```python
from build123d import *

# Parameters (mm, degrees)
CUT_EXTRUDE_1_REACH = 159.944
SKETCH_2_R          = 2.15


with BuildPart() as part:
    # 草图1 → 旋转1 (revolve)
    with BuildSketch(Plane.XY, mode=Mode.PRIVATE) as revolve_1_sk:
        Polygon((111.6, 6.1), (111.6, 8.1), (109.6, 8.1), (109.6, 6.1), (96.1, 6.1), (96.1, 0), (111.6, 0), align=None)
    revolve(revolve_1_sk.sketch.rotate(Axis((0, 0, 0), (0, 1, 0)), 90), axis=Axis((0, 0, 0), (0, 1, 0)))

    # 草图2 → 切除-拉伸1 (cut, up to next)
    with BuildSketch(Plane(origin=(0, 6.1, 0), x_dir=(1, 0, 0), z_dir=(0, 1, 0)), mode=Mode.PRIVATE) as cut_extrude_1_sk1:
        with Locations(Location((-100.25, 0, 0), (0, 0, 270))):
            Circle(SKETCH_2_R)
    cut_extrude_1_tool1 = extrude(cut_extrude_1_sk1.sketch, amount=-CUT_EXTRUDE_1_REACH, mode=Mode.PRIVATE) & part.part
    # 草图2 → 切除-拉伸1 (cut, up to next)
    with BuildSketch(Plane(origin=(0, 6.1, 0), x_dir=(1, 0, 0), z_dir=(0, 1, 0)), mode=Mode.PRIVATE) as cut_extrude_1_sk2:
        with Locations(Location((-70.887454814, 70.887454814, 0), (0, 0, 270))):
            Circle(SKETCH_2_R)
    cut_extrude_1_tool2 = extrude(cut_extrude_1_sk2.sketch, amount=-CUT_EXTRUDE_1_REACH, mode=Mode.PRIVATE) & part.part
    # 草图2 → 切除-拉伸1 (cut, up to next)
    with BuildSketch(Plane(origin=(0, 6.1, 0), x_dir=(1, 0, 0), z_dir=(0, 1, 0)), mode=Mode.PRIVATE) as cut_extrude_1_sk3:
        with Locations(Location((0, 100.25, 0), (0, 0, 270))):
            Circle(SKETCH_2_R)
    cut_extrude_1_tool3 = extrude(cut_extrude_1_sk3.sketch, amount=-CUT_EXTRUDE_1_REACH, mode=Mode.PRIVATE) & part.part
    # 草图2 → 切除-拉伸1 (cut, up to next)
    with BuildSketch(Plane(origin=(0, 6.1, 0), x_dir=(1, 0, 0), z_dir=(0, 1, 0)), mode=Mode.PRIVATE) as cut_extrude_1_sk4:
        with Locations(Location((70.887454814, 70.887454814, 0), (0, 0, 270))):
            Circle(SKETCH_2_R)
    cut_extrude_1_tool4 = extrude(cut_extrude_1_sk4.sketch, amount=-CUT_EXTRUDE_1_REACH, mode=Mode.PRIVATE) & part.part
    # 草图2 → 切除-拉伸1 (cut, up to next)
    with BuildSketch(Plane(origin=(0, 6.1, 0), x_dir=(1, 0, 0), z_dir=(0, 1, 0)), mode=Mode.PRIVATE) as cut_extrude_1_sk5:
        with Locations(Location((100.25, 0, 0), (0, 0, 270))):
            Circle(SKETCH_2_R)
    cut_extrude_1_tool5 = extrude(cut_extrude_1_sk5.sketch, amount=-CUT_EXTRUDE_1_REACH, mode=Mode.PRIVATE) & part.part
    # 草图2 → 切除-拉伸1 (cut, up to next)
    with BuildSketch(Plane(origin=(0, 6.1, 0), x_dir=(1, 0, 0), z_dir=(0, 1, 0)), mode=Mode.PRIVATE) as cut_extrude_1_sk6:
        with Locations(Location((70.887454814, -70.887454814, 0), (0, 0, 270))):
            Circle(SKETCH_2_R)
    cut_extrude_1_tool6 = extrude(cut_extrude_1_sk6.sketch, amount=-CUT_EXTRUDE_1_REACH, mode=Mode.PRIVATE) & part.part
    # 草图2 → 切除-拉伸1 (cut, up to next)
    with BuildSketch(Plane(origin=(0, 6.1, 0), x_dir=(1, 0, 0), z_dir=(0, 1, 0)), mode=Mode.PRIVATE) as cut_extrude_1_sk7:
        with Locations(Location((0, -100.25, 0), (0, 0, 270))):
            Circle(SKETCH_2_R)
    cut_extrude_1_tool7 = extrude(cut_extrude_1_sk7.sketch, amount=-CUT_EXTRUDE_1_REACH, mode=Mode.PRIVATE) & part.part
    # 草图2 → 切除-拉伸1 (cut, up to next)
    with BuildSketch(Plane(origin=(0, 6.1, 0), x_dir=(1, 0, 0), z_dir=(0, 1, 0)), mode=Mode.PRIVATE) as cut_extrude_1_sk8:
        with Locations(Location((-70.887454814, -70.887454814, 0), (0, 0, 270))):
            Circle(SKETCH_2_R)
    cut_extrude_1_tool8 = extrude(cut_extrude_1_sk8.sketch, amount=-CUT_EXTRUDE_1_REACH, mode=Mode.PRIVATE) & part.part
    add(cut_extrude_1_tool1.solids().sort_by_distance((-100.25, 6.1, 0))[0], mode=Mode.SUBTRACT)
    add(cut_extrude_1_tool2.solids().sort_by_distance((-70.887455, 6.1, -70.887455))[0], mode=Mode.SUBTRACT)
    add(cut_extrude_1_tool3.solids().sort_by_distance((0, 6.1, -100.25))[0], mode=Mode.SUBTRACT)
    add(cut_extrude_1_tool4.solids().sort_by_distance((70.887455, 6.1, -70.887455))[0], mode=Mode.SUBTRACT)
    add(cut_extrude_1_tool5.solids().sort_by_distance((100.25, 6.1, 0))[0], mode=Mode.SUBTRACT)
    add(cut_extrude_1_tool6.solids().sort_by_distance((70.887455, 6.1, 70.887455))[0], mode=Mode.SUBTRACT)
    add(cut_extrude_1_tool7.solids().sort_by_distance((0, 6.1, 100.25))[0], mode=Mode.SUBTRACT)
    add(cut_extrude_1_tool8.solids().sort_by_distance((-70.887455, 6.1, 70.887455))[0], mode=Mode.SUBTRACT)


solid = part.part
```
CAD build for the part. Positions are in the model's coordinates, mm. A direction names the side the tool comes from. Round coordinates to 2 decimals unless told otherwise and drop trailing zeros. Write each loop counter-clockwise with the first axis right and the second up, starting at its lowest first coordinate (ties: lowest second). Pieces come first, ordered by that corner, then holes. Notation, with made-up numbers: (-33.5, -33) - (8.5, -33) arc R28 ccw to (8.5, -8) - close; hole circle Ø3 at (0.25, -37). An arc over 180 degrees is marked (long way). Write item = value, one per line. Start each with the question number.
Q1. Probe L1, parallel to X at y = 7.1, z = 0; L2, parallel to X at y = 1.5, z = 0.5; L3, parallel to Z at x = 26.5, y = 7.5. List the from-to ranges inside material, lowest first. Write a range as from..to.
Q2. Which spindle directions (+Z, -Z, +X, -X, +Y, -Y) get a long thin tool onto all of the face, cutting with end or side? Do faces 1 (the cylindrical face through (-74.07, 7.09, 80.78)), 2 (the cylindrical face through (-28.87, 3.01, -91.66)). Say none if no direction does.
Q3. Mould opens along X. For faces 3 (the flat face through (97, 6.1, 1)), 4 (the cylindrical face through (108.946, 4.107, 24.193)), 5 (the flat face through (74, 8.1, -82)) say: pulls with the +X half, pulls with the -X half, needs draft (parallel to the pull), parting line crosses it, or undercut.
Q4. Band-saw the part on B-B (x = -77). Give the cut face in (y, z).
Q5. Drop flat-ended pins along their axis: pin 1 (3 mm diameter, centred on y = 2, z = -60.5, fed in from -X); pin 2 (7 mm diameter, centred on x = -100.25, z = 0, fed in from +Y); pin 3 (1.5 mm diameter, centred on y = 3.5, z = 10.5, fed in from -X). Give the stop position or say it passes through.
Q6. Band-saw the part on A-A (z = -36.5). Give the cut face in (x, y), then the cut area to 3 significant figures.
Q7. Band-saw the part on C-C (y = 4.5). Count the separate pieces of the cut face and the enclosed holes in it, then the cut area to 4 significant figures.
Answers below:
q1.L1 = -111.6..-109.6, 109.6..111.6
q1.L2 = -111.6..-102.34, -98.16..-96.1, 96.1..98.16, 102.34..111.6
q1.L3 = -108.41..-106.35, 106.35..108.41
q2.face_1 = +Y
q2.face_2 = +Y, -Y
q3.face_3 = undercut
q3.face_4 = parting line crosses it
q3.face_5 = needs draft
q4.outline = (0, -80.78) - (8.1, -80.78) - (8.1, -77.99) - (6.1, -77.99) - (6.1, -57.5) - (0, -57.5) - close; (0, 57.5) - (6.1, 57.5) - (6.1, 77.99) - (8.1, 77.99) - (8.1, 80.78) - (0, 80.78) - close
q5.pin_1 = -94.73
q5.pin_2 = 6.1
q5.pin_3 = -111.17
q6.outline = (-105.46, 0) - (-88.9, 0) - (-88.9, 6.1) - (-103.34, 6.1) - (-103.34, 8.1) - (-105.46, 8.1) - close; (88.9, 0) - (105.46, 0) - (105.46, 8.1) - (103.34, 8.1) - (103.34, 6.1) - (88.9, 6.1) - close
q6.area = 211 mm2
q7.separate_pieces = 1
q7.enclosed_holes = 9
q7.area = 10,000 mm2
